Can you work these out from the model? Positions are in its coordinate system, mm. Face numbers are marked on the shaded views. A direction names the side the tool comes from. Round coordinates to 2 decimals unless told otherwise and drop trailing zeros. Loops run counter-clockwise (first coordinate to the right, second up) from the corner with the lowest first, then second, coordinate; pieces in that order, holes last. Notation, with made-up numbers: M 64,74.5 L 101,74.5 A25 cw 101,106.5 Z; hole C -25,68.25 d8. An arc over 180 degrees is marked long. Use a Markdown table: item, result. Add a question column.
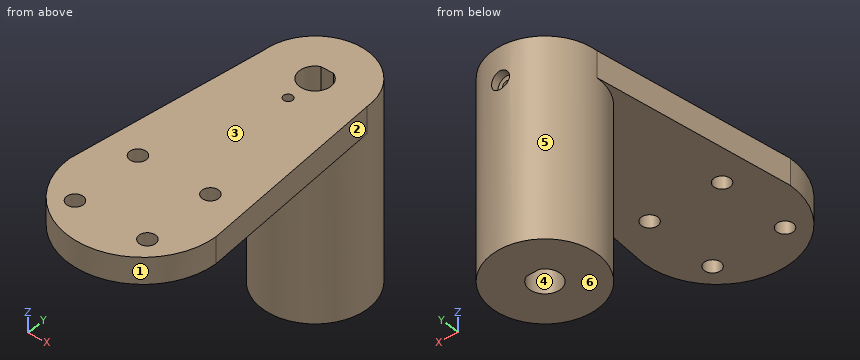
Autodesk Inventor part; units mm, degrees
ref_plane "Work Plane2" through (1, 76, 8) normal (0, 1, 0) x (-1, 0, 0)
ref_plane "YZ Plane" through (0, 0, 0) normal (1, 0, 0) x (0, 1, 0)
ref_plane "XZ Plane" through (0, 0, 0) normal (0, 1, 0) x (-1, 0, 0)
sketch "Sketch1" plane through (0, 0, 0) normal (0, 0, 1) x (1, 0, 0)
  arc A0 (-22.5, 0) -> (22.5, 0) centre (0, 0) ccw
  circle A1 centre (-11.1871, 11.1871) radius 2.5
  arc A2 (17, 60) -> (-15, 60) centre (1, 60) ccw
  line L0 (22.5, 0) -> (17, 60)
  line L1 (-22.5, 0) -> (-15, 60)
  circle A3 centre (11.0869, 11.1871) radius 2.5
  line L2 (-1.4379, 0) -> (3.0127, 0) construction
  circle A4 centre (-11.1871, -11.1871) radius 2.5
  circle A5 centre (11.0869, -11.1871) radius 2.5
  dimension "d0" = 45
  dimension "d3" = 5
  dimension "d29" = 32
  dimension "d57" = 5
  dimension "d58" = 22.274
  dimension "d59" = 15.821
extrude "Extrusion1" add sketch "Sketch1" along normal blind 8
sketch "Sketch5" plane through (0, 0, 8) normal (0, 0, 1) x (1, 0, 0)
  arc A0 (17, 60) -> (-15, 60) centre (1, 60) ccw
  circle A1 centre (1, 60) radius 16
  point P0 (0, 0)
  point P1 (-15, 60)
  dimension "d44" = 32
extrude "Extrusion3" add sketch "Sketch5" against normal blind 60
sketch "Sketch6" plane through (0, 0, 8) normal (0, 0, 1) x (1, 0, 0)
  arc A0 (17, 60) -> (-15, 60) centre (1, 60) ccw
  arc A1 (-0.9268, 64.2869) -> (2.9268, 64.2869) centre (1, 60) ccw
  line L0 (-0.9268, 64.2869) -> (2.9268, 64.2869)
  point P0 (0, 0)
  point P1 (1, 55.3)
  point P2 (1, 64.2869)
  dimension "d32" = 9.4
  dimension "d43" = 4.2869
extrude "Extrusion4" cut sketch "Sketch6" against normal through all
ref_plane "Work Plane2" through (1, 76, 8) normal (0, 1, 0) x (-1, 0, 0)
sketch "Sketch9" plane through (1, 76, 8) normal (0, 1, 0) x (-1, 0, 0)
  line L0 (16, 0) -> (-16, 0)
  line L1 (0, 0) -> (0, -10)
  circle A0 centre (0, -10) radius 1.35
  point P0 (1, -8)
  dimension "d45" = 10
  dimension "d46" = 2.7
extrude "Extrusion7" cut sketch "Sketch9" against normal blind 12
sketch "Sketch10" plane through (1, 76, 8) normal (0, 1, 0) x (-1, 0, 0)
  circle A0 centre (0, -10) radius 1.35
  circle A1 centre (0, -10) radius 2.75
  point P0 (1, -8)
  dimension "d49" = 5.5
extrude "Extrusion8" cut sketch "Sketch10" against normal blind 2.5
sketch "Sketch13" plane through (0, 0, 8) normal (0, 0, 1) x (1, 0, 0)
  circle A0 centre (1, 50.438) radius 1.4
  arc A1 (-0.9268, 64.2869) -> (2.9268, 64.2869) centre (1, 60) ccw
  point P0 (0, 0)
  dimension "d60" = 2.8
  dimension "d61" = 9.562
extrude "Extrusion11" cut sketch "Sketch13" against normal blind 15
properties part number "pen_holder" material "LCP Plastic"
(1) On a 3-axis mill with a long thin cutter (end or side, diameter ignored), from which of +Z, -Z, +X, -X, +Y, -Y can I reach the whole of each face in a straight line? I mean the marked faces 5 and 6. Say none if no direction works.
(2) Suppose I cut it at B-B on z = -36. List the corners of the cut face in (x, y) for me.
(3) Thinking about a two-plate mould opening in X: for the marked faces 1, 2, 3 and 4, which applies, released by +X, released by -X, zero draft, split by the parting line, or undercut?
(4) If I drill on probe 1 along X at (y, z) = (60, -19); probe 2 along Z at (x, y) = (1, 68.75); probe 3 along Z at (x, y) = (14.5, 46.5), over which ranges is the centre line in solid material (lowest first)? Write a range as [from, to].
(5) I'm going to push flat-ended pins straight in: pin 1 (4.5 mm diameter, centred on x = -11.19, y = -11.19, fed in from +Z); pin 2 (5 mm diameter, centred on x = 1, z = -2, fed in from +Y); pin 3 (12 mm diameter, centred on y = 46.5, z = -37, fed in from +X); pin 4 (1.5 mm diameter, centred on x = -5, z = -18.5, fed in from -Y). Where does each tip first touch, or does it pass through?
(6) Suppose I cut it at D-D on z = 2. List the corners of the cut face in (x, y) for me, and give its area (3 significant figures).
(7) Suppose I cut it at C-C on y = 65.5. List the corners of the cut face in (x, z) for me.
(8) Suppose I cut it at A-A on x = 1. List the corners of the cut face in (y, z) for me, and give its area (3 significant figures).
Results below:
| question | item | result |
|---|---|---|
| 1 | face 5 | -Z |
| 1 | face 6 | -Z, +X, -X, +Y, -Y |
| 2 | outline | C 1,60 d32; hole M -0.93,64.29 A4.7 ccw long 2.93,64.29 Z |
| 3 | face 1 | split by the parting line |
| 3 | face 2 | released by +X |
| 3 | face 3 | zero draft |
| 3 | face 4 | undercut |
| 4 | probe 1 | x = [-15, -3.7], [5.7, 17] |
| 4 | probe 2 | z = [-52, -3.35], [-0.65, 8] |
| 4 | probe 3 | z = [0, 8] |
| 5 | pin 1 | passes through |
| 5 | pin 2 | stops at y = 73.5 |
| 5 | pin 3 | stops at x = 15.13 |
| 5 | pin 4 | stops at y = 44.89 |
| 6 | outline | M -22.5,0 A22.5 ccw 22.5,0 L 17,60 A16 ccw -15,60 Z; hole C -11.19,-11.19 d5; hole C -11.19,11.19 d5; hole M -0.93,64.29 A4.7 ccw long 2.93,64.29 Z; hole C 1,50.44 d2.8; hole C 11.09,-11.19 d5; hole C 11.09,11.19 d5 |
| 6 | area | 3,350 mm² |
| 7 | outline | M -14.02,-52 L 16.02,-52 L 16.02,8 L -14.02,8 Z; hole C 1,-2 d2.7 |
| 8 | outline | M -22.48,0 L 44,0 L 44,-52 L 55.3,-52 L 55.3,8 L 51.84,8 L 51.84,-7 L 49.04,-7 L 49.04,8 L -22.48,8 Z; M 64.29,-52 L 76,-52 L 76,-4.75 L 73.5,-4.75 L 73.5,-3.35 L 64.29,-3.35 Z; M 64.29,-0.65 L 73.5,-0.65 L 73.5,0.75 L 76,0.75 L 76,8 L 64.29,8 Z |
| 8 | area | 1,830 mm² |
